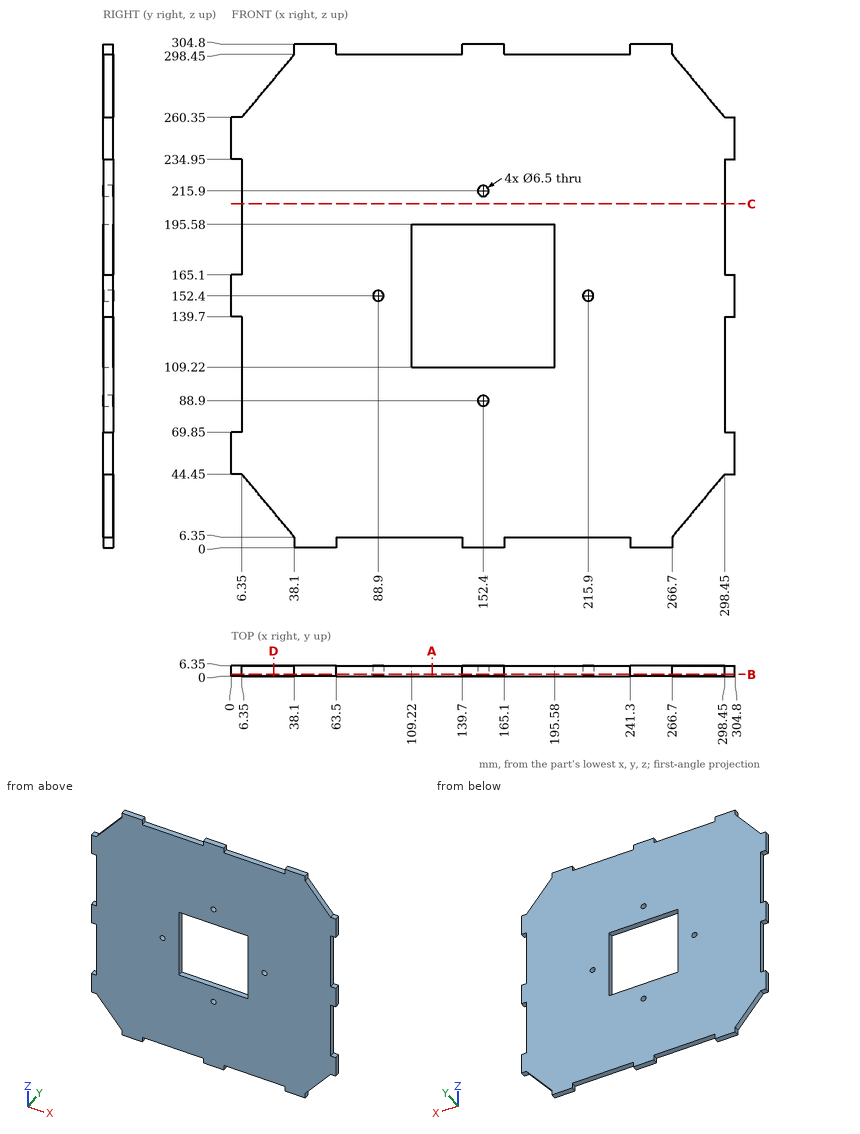
Can you work these out from the drawing? Everything is in mm from the part's minimum corner. Give positions to 0.01 mm unless a question says otherwise; leave off trailing zeros. Order: outer loops, then holes, each group sorted by start corner. A loop starts at its lowest first (then second) coordinate and runs counter-clockwise, first axis right, second up.
Item 1: If we section it at B-B, the plane y = 1: Count the separate pieces of the cut face and the enclosed holes in it, plus the area to 3 significant figures.
Item 2: I need wall thicknesses on line 1 (Z direction, x = 152.4, y = 2.5); line 2 (Z direction, x = 117, y = 4.75); line 3 (X direction, y = 4.5, z = 215.9). Which ranges of each line are inside material? Lowest first, please.
Item 3: If we section it at A-A, the plane x = 121.5: Write out the boundary of the cut face in (y, z).
Item 4: If we section it at C-C, the plane z = 208: Write out the boundary of the cut face in (x, y), plus the area to 3 significant figures.
Item 5: I'm going to push flat-ended pins straight in: pin 1 (2 mm diameter, centred on y = 2.5, z = 88, fed in from -X); pin 2 (2 mm diameter, centred on y = 1.5, z = 230, fed in from +X); pin 3 (1.9 mm diameter, centred on x = 301, y = 2, fed in from -Z). Where does each tip first touch, or does it pass through?
Item 6: If we section it at D-D, the plane x = 25.5: Write out the boundary of the cut face in (y, z).
Values:
1. separate pieces: 1
1. enclosed holes: 5
1. area: 77,200 mm2
2. line 1: z = 0 to 85.65, 92.15 to 109.22, 195.58 to 212.65, 219.15 to 304.8
2. line 2: z = 6.35 to 109.22, 195.58 to 298.45
2. line 3: x = 6.35 to 149.15, 155.65 to 298.45
3. outline: (0, 6.35) - (6.35, 6.35) - (6.35, 109.22) - (0, 109.22) - close; (0, 195.58) - (6.35, 195.58) - (6.35, 298.45) - (0, 298.45) - close
4. outline: (6.35, 0) - (298.45, 0) - (298.45, 6.35) - (6.35, 6.35) - close
4. area: 1,850 mm2
5. pin 1: stops at x = 6.35
5. pin 2: stops at x = 298.45
5. pin 3: stops at z = 44.45
6. outline: (0, 21.47) - (6.35, 21.47) - (6.35, 283.33) - (0, 283.33) - close
